Verification items for the finished model (mm, model axes). A direction names the side the tool comes from. Round coordinates to 2 decimals unless told otherwise and drop trailing zeros. Order: outer loops, then holes, each group sorted by start corner. A loop starts at its lowest first (then second) coordinate and runs counter-clockwise, first axis right, second up. Notation, with made-up numbers: M -6,88 L -1,88 A33 ccw -1,126 Z; hole C -36,-14 d9. An arc over 180 degrees is marked long. Use CSV: the item, a comma, the result in double quotes. Start each with the question number.
Q1. Set-up check for faces 4 (the face through (0, -1, 7)), 5 (the face through (12, 16, -49)): record each of +Z, -Z, +X, -X, +Y, -Y from which the full face is reachable in a straight line by a thin tool's end or side.
Q2. Sectioned sample at A-A (z = 83). Enter the section's corners in (x, y), and give its area (3 significant figures).
Q3. Mould release check, pull along Z, two halves, no side actions. Record for faces 1 (the face through (5.92, -2.15, 99.36)), 2 (the face through (7, -1, 125)), 3 (the face through (7, -60, 3)): +Z half, -Z half, draft (parallel to the pull), parting line (faces both ways), or undercut.
Q4. Sectioned sample at D-D (z = -4). Enter the section's corners in (x, y).
Q5. Sectioned sample at C-C (z = -32.5). Enter the section's corners in (x, y), and give its area (3 significant figures).
Q6. Gauge pin test, flat ends, axial feed: pin 1 Ø4.5 at (y, z) = (50, 117) entering from -X; pin 2 Ø4 at (y, z) = (-21.57, -54.07) entering from +X. Record the tip position at first contact, or that the pin passes through.
Q7. Sectioned sample at B-B (x = 5). State how many separate pieces and enclosed holes the cut face has, and give its area (3 significant figures).
Q8. Scan lines: line 1 (Z direction, x = 5.25, y = 0); line 2 (Z direction, x = 4.25, y = 21); line 3 (Z direction, x = 4.25, y = 7). Record each from-to range of solid material in increasing order.
```python
from build123d import *

# Parameters (mm, degrees)
F0_W     = 120
F0_H     = 240
F0_R     = 2
F0_R_2   = 37.5
F0_R_3   = 22
F1_DEPTH = 15
F0_R_4   = 16.5
F0_R_5   = 1.5
F0_R_6   = 22.75
F2_DEPTH = 12


with BuildPart() as f1:
    # F0 (on Right) → F1 (new body)
    with BuildSketch(Plane.YZ):
        with Locations((0, 5)):
            Rectangle(F0_W, F0_H)
        with Locations((-49.999999, -107)):
            Circle(F0_R, mode=Mode.SUBTRACT)
        with Locations((50.000001, -107)):
            Circle(F0_R, mode=Mode.SUBTRACT)
        with Locations((0, -32.5)):
            Circle(F0_R_2, mode=Mode.SUBTRACT)
        with Locations((-49.999999, 117)):
            Circle(F0_R, mode=Mode.SUBTRACT)
        with Locations((0, 83)):
            Circle(F0_R_3, mode=Mode.SUBTRACT)
        with Locations((50.000001, 117.000003)):
            Circle(F0_R, mode=Mode.SUBTRACT)
    extrude(amount=F1_DEPTH)

    # F0 (on Right) → F2 (join)
    with BuildSketch(Plane.YZ):
        with Locations((0, 83)):
            Circle(F0_R_3)
        with Locations((0, 83)):
            Circle(F0_R_4, mode=Mode.SUBTRACT)
        with Locations((0, -32.5)):
            Circle(F0_R_2)
        with Locations((-21.566757, -54.066757)):
            Circle(F0_R_5, mode=Mode.SUBTRACT)
        with Locations((-21.566757, -10.933243)):
            Circle(F0_R_5, mode=Mode.SUBTRACT)
        with Locations((0, -32.5)):
            Circle(F0_R_6, mode=Mode.SUBTRACT)
        with Locations((21.566757, -54.066757)):
            Circle(F0_R_5, mode=Mode.SUBTRACT)
        with Locations((21.566757, -10.933243)):
            Circle(F0_R_5, mode=Mode.SUBTRACT)
    extrude(amount=F2_DEPTH)


solid = f1.part
```
Verdict:
1,face 4,"+Z, -Z, -X, +Y, -Y"
1,face 5,"+X"
2,outline,"M 0,-60 L 15,-60 L 15,-22 L 12,-22 L 12,-16.5 L 0,-16.5 Z; M 0,16.5 L 12,16.5 L 12,22 L 15,22 L 15,60 L 0,60 Z"
2,area,"1,270 mm²"
3,face 1,"undercut"
3,face 2,"+Z half"
3,face 3,"draft"
4,outline,"M 0,-60 L 15,-60 L 15,-24.37 L 12,-24.37 L 12,24.37 L 15,24.37 L 15,60 L 0,60 Z"
5,outline,"M 0,-60 L 15,-60 L 15,-37.5 L 12,-37.5 L 12,-22.75 L 0,-22.75 Z; M 0,22.75 L 12,22.75 L 12,37.5 L 15,37.5 L 15,60 L 0,60 Z"
5,area,"1,030 mm²"
6,pin 1,"stops at x = 0"
6,pin 2,"stops at x = 12"
7,separate pieces,"1"
7,enclosed holes,"10"
7,area,"26,200 mm²"
8,line 1,"z = -115 to -55.25, -9.75 to 66.5, 99.5 to 125"
8,line 2,"z = -115 to -55.46, -52.68 to -41.25, -23.75 to -12.32, -9.54 to 125"
8,line 3,"z = -115 to -54.15, -10.85 to 68.06, 97.94 to 125"
